The drawing under review shows one solid part. Ordinate dimensions are in mm from its lowest x, y, z. A direction names the side the tool comes from. Round coordinates to 2 decimals unless told otherwise and drop trailing zeros. Order: outer loops, then holes, each group sorted by start corner. A loop starts at its lowest first (then second) coordinate and runs counter-clockwise, first axis right, second up. Notation, with made-up numbers: (78, 52.5) -> (96, 52.5) arc R16 cw to (96, 63.5) -> close; hole circle Ø11 at (2, 36.5). An arc over 180 degrees is marked (long way). Return JSON: item names as keys, results as strings. Group by question number.
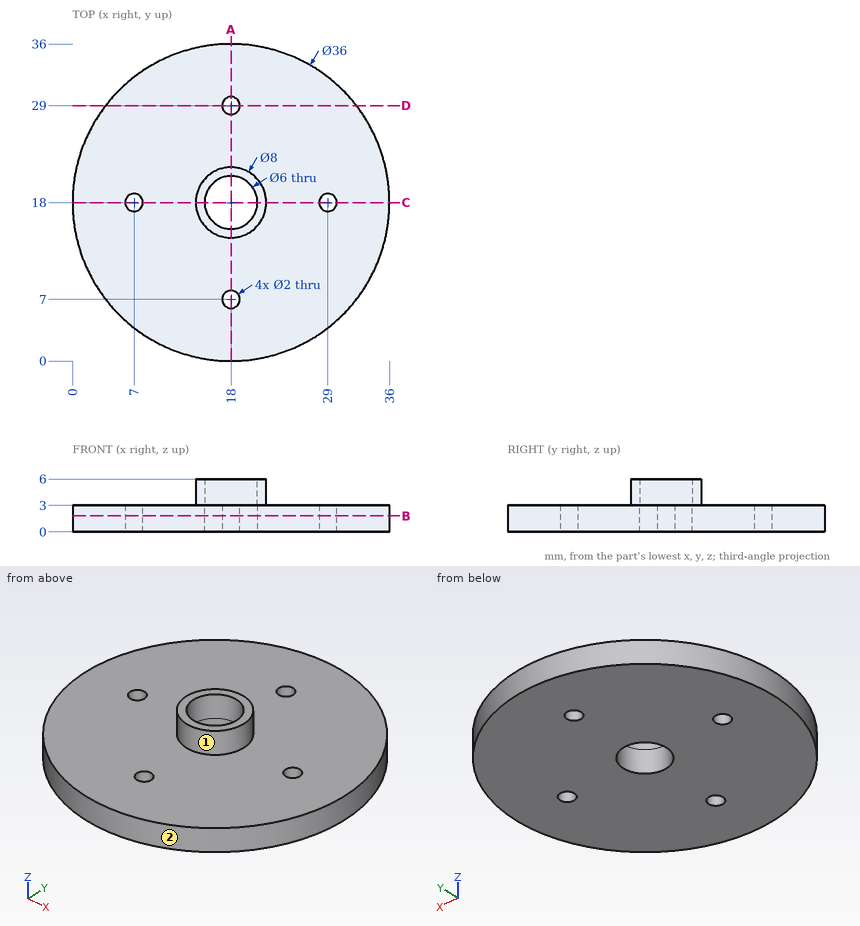
Item 1: Consider section D-D on y = 29. State the section outline as (x, z) points.
Item 2: Consider section B-B on z = 1.8. State the section outline as (x, y) points, plus the area to 3 significant figures.
Item 3: Wall thickness on line 1 along Y through (x, z) = (18, 2); line 2 along Y through (x, z) = (18, 3.75); line 3 along Z through (x, y) = (9.5, 20): over which ranges is each line inside the solid? List them lowest first.
Item 4: Insertion check: pin 1 Ø10 at (x, y) = (5.5, 29) entering from -Z; pin 2 Ø1 at (x, y) = (29, 9) entering from +Z; pin 3 Ø1.5 at (x, z) = (13.5, 0.5) entering from -Y; pin 4 Ø3 at (x, z) = (28, 2.5) entering from -Y. Each pin has a flat end and moves straight along its axis. Give the tip position at first contact, or say it passes through.
Item 5: For the marked faces 1 and 2, list the 3-axis set-ups (+Z, -Z, +X, -X, +Y, -Y) from which the entire face can be reached by the end or side of a thin tool; tool diameter is ignored.
Item 6: Consider section A-A on x = 18. State the section outline as (y, z) points.
Values:
{
 "1": {"outline": "(3.75, 0) -> (17, 0) -> (17, 3) -> (3.75, 3) -> close; (19, 0) -> (32.25, 0) -> (32.25, 3) -> (19, 3) -> close"},
 "2": {"outline": "circle Ø36 at (18, 18); hole circle Ø2 at (7, 18); hole circle Ø6 at (18, 18); hole circle Ø2 at (18, 7); hole circle Ø2 at (18, 29); hole circle Ø2 at (29, 18)", "area": "977 mm^2"},
 "3": {"line 1": "0 to 6, 8 to 15, 21 to 28, 30 to 36", "line 2": "14 to 15, 21 to 22", "line 3": "0 to 3"},
 "4": {"pin 1": "z = 0", "pin 2": "z = 3", "pin 3": "y = 0.39", "pin 4": "y = 2.13"},
 "5": {"face 1": "+Z", "face 2": "+Z, -Z"},
 "6": {"outline": "(0, 0) -> (6, 0) -> (6, 3) -> (0, 3) -> close; (8, 0) -> (15, 0) -> (15, 6) -> (14, 6) -> (14, 3) -> (8, 3) -> close; (21, 0) -> (28, 0) -> (28, 3) -> (22, 3) -> (22, 6) -> (21, 6) -> close; (30, 0) -> (36, 0) -> (36, 3) -> (30, 3) -> close"}
}
